```python
from build123d import *

# Parameters (mm, degrees)
BASPROSKE_W           = 12
BASPROSKE_H           = 22
TOOTHCUT_DEPTH        = 34.346664001
TEETHCUTS_COUNT       = 20
TEETHCUTS_ANGLE       = 342
BORSKE_R              = 0.4
BORE_DEPTH            = 50.0000508
KES_EKSTR_ZYON1_DEPTH = 100


with BuildPart() as part:
    # BasProSke → Base-Revolve (revolve)
    with BuildSketch(Plane(origin=(0, 0, 0), x_dir=(1, 0, 0), z_dir=(0, 1, 0)), mode=Mode.PRIVATE) as base_revolve_sk:
        with Locations((6, 11)):
            Rectangle(BASPROSKE_W, BASPROSKE_H)
    revolve(base_revolve_sk.sketch.rotate(Axis((-10, 0, 0), (1, 0, 0)), 180), axis=Axis((-10, 0, 0), (1, 0, 0)))

    # TooCutSke → ToothCut (cut, through all)
    with BuildSketch(Plane(origin=(0, 0, 0), x_dir=(0, 0, -1), z_dir=(1, 0, 0))):
        with BuildLine():
            ThreePointArc((0.986171591, 17.471189616), (0, 17.499), (-0.986171591, 17.471189616))
            ThreePointArc((-0.986171591, 17.471189616), (-1.626916196, 19.798789858), (-2.932850173, 21.829260982))
            ThreePointArc((-2.932850173, 21.829260982), (0, 22.0254), (2.932850173, 21.829260982))
            ThreePointArc((2.932850173, 21.829260982), (1.626916196, 19.798789858), (0.986171591, 17.471189616))
        make_face()
    toothcut = extrude(amount=TOOTHCUT_DEPTH, mode=Mode.SUBTRACT)

    # TeethCuts: ToothCut ×20 about axis
    teethcuts_axis = Axis((-10, 0, 0), (1, 0, 0))
    for i in range(1, TEETHCUTS_COUNT):
        add(toothcut.rotate(teethcuts_axis, i * TEETHCUTS_ANGLE / (TEETHCUTS_COUNT - 1)), mode=Mode.SUBTRACT)

    # BorSke → Bore (cut, symmetric)
    with BuildSketch(Plane(origin=(0, 0, 0), x_dir=(0, 0, -1), z_dir=(1, 0, 0))):
        with Locations(Location((0, 0, 0), (0, 0, 180))):
            Circle(BORSKE_R)
    extrude(amount=BORE_DEPTH, both=True, mode=Mode.SUBTRACT)

    # Çizim1 → Kes-Ekstrüzyon1 (cut)
    with BuildSketch(Plane(origin=(12, 0, 0), x_dir=(0, 0, -1), z_dir=(1, 0, 0))):
        with BuildLine():
            ThreePointArc((3.105, 0), (0.947725377, 2.956829655), (-2.526459974, 1.805))
            Line((-2.526459974, 1.805), (-2.526459974, -1.805))
            ThreePointArc((-2.526459974, -1.805), (0.947725377, -2.956829655), (3.105, 0))
        make_face()
    extrude(amount=-KES_EKSTR_ZYON1_DEPTH, mode=Mode.SUBTRACT)


solid = part.part
```
Geometry: final body of the model. Coordinates: model frame, mm. A direction names the side the tool comes from. Coordinates: 2 decimals unless noted, no trailing zeros. Write each loop counter-clockwise with the first axis right and the second up, starting at its lowest first coordinate (ties: lowest second). Pieces come first, ordered by that corner, then holes. Notation, with made-up numbers: M 8.25,8.25 L 65.25,8.25 A13 ccw 65.25,31.25 Z; hole C -26.5,38 d4. An arc over 180 degrees is marked long. Use CSV: the item, a comma, the result in double quotes. Start each with the question number.
1. Reachability of faces 1 (the face through (5.916, 12.911, -15.037)), 2 (the face through (5.92, -14.17, -10.27)), 3 (the face through (5.916, 7.678, 18.341)), 4 (the face through (5.916, 19.754, 1.607)) from +Z, -Z, +X, -X, +Y, -Y: full face, straight path, thin tool, end or side. Return the list, or none.
2. Cut plane A-A on z = -12.5. Return the cut outline in (x, y).
3. Cut plane B-B on y = -12. Return the cut outline in (x, z), plus the area to 3 significant figures.
4. Ray query, probe 1 along Z at (x, y) = (5, -14.5); probe 2 along Z at (x, y) = (8.5, 19). Return the intervals inside material, ascending.
5. Mould query, pull axis Y, two halves, no side actions, for faces 5 (the face through (6.084, -9.981, 19.606)), 6 (the face through (5.916, -10.297, -14.149)), 7 (the face through (5.9, 17.5, 0)). Classes: pulls with the +Y half, pulls with the -Y half, needs draft (parallel to the pull), parting line crosses it, or undercut.
6. First-contact query: P1, Ø1.5, axis at x = 10, y = 14, coming from the +Z side; P2, Ø4, axis at x = 1.5, y = -4.5, coming from the -Z side; P3, Ø6, axis at x = 5, y = -15, coming from the +Z side. Flat tips, straight axial feed; report the tip coordinate or a pass-through.
Entries:
1,face 1,"-Z, +X, -X"
1,face 2,"+X, -X"
1,face 3,"+Z, +X, -X"
1,face 4,"+X, -X, +Y"
2,outline,"M 0,-14.78 L 12,-14.78 L 12,14.78 L 0,14.78 Z"
3,outline,"M 0,-14.42 L 12,-14.42 L 12,14.42 L 0,14.42 Z"
3,area,"346 mm²"
4,probe 1,"-15.75 to -12.11, -9.8 to 9.8, 12.11 to 15.75"
4,probe 2,"-10.49 to -8.35, -4.6 to -1.32, 1.32 to 4.6, 8.35 to 10.49"
5,face 5,"pulls with the -Y half"
5,face 6,"undercut"
5,face 7,"pulls with the +Y half"
6,P1,"z = 15.82"
6,P2,"z = -21.81"
6,P3,"z = 15.93"
